Source: CAD feature listing. Evaluate the final solid. Frame: model axes, mm. A direction names the side the tool comes from. Round coordinates to 2 decimals unless told otherwise and drop trailing zeros. Loops run counter-clockwise (first coordinate to the right, second up) from the corner with the lowest first, then second, coordinate; pieces in that order, holes last.
(1) Section C-C, the plane y = 4.5. Return the cut outline in (x, z) (3 decimals), plus the area to 3 significant figures.
(2) Section A-A, the plane x = 0. Return the cut outline in (y, z), plus the area to 3 significant figures.
(3) Mould query, pull axis X, two halves, no side actions, for faces 1 (the flat face through (7, 0, -7)), 2 (the cylindrical face through (-9.874, 8.535, -9.663)), 3 (the cylindrical face through (9.777, 9.042, 9.758)). Classes: pulls with the +X half, pulls with the -X half, needs draft (parallel to the pull), parting line crosses it, or undercut.
(4) Material intervals for probe 1 along X at (y, z) = (8.2, 0); probe 2 along Y at (x, z) = (-0.75, -9); probe 3 along Z at (x, y) = (-14.75, 9), sorted ascending.
(5) Section B-B, the plane y = 10.25. Return the cut outline in (x, z).
(6) First-contact query: pin 1 Ø10 at (x, z) = (3.5, 0) entering from +Y; pin 2 Ø6 at (y, z) = (2.5, -9) entering from +X; pin 3 Ø9 at (x, z) = (0, 0) entering from -Y. Flat tips, straight axial feed; report the tip coordinate or a pass-through.
(7) Set-up query: faces 4 (the conical face through (-13.585, 11.16, 7.574)), 5 (the cylindrical face through (-5.776, 3.042, -8.602)). Return all of +Z, -Z, +X, -X, +Y, -Y with unobstructed straight access to the full face (end or side cutting, diameter ignored); none if empty.
```python
from build123d import *

# Parameters (mm, degrees)
SKETCH1_W                   = 21
SKETCH1_H                   = 21
BOSS_EXTRUDE1_DEPTH         = 12
CUT_EXTRUDE1_REACH          = 21.092
SKETCH2_R                   = 7.4
SKETCH3_W                   = 21
SKETCH3_H                   = 6
BOSS_EXTRUDE2_DEPTH         = 8.99
SKETCH4_W                   = 21
SKETCH4_H                   = 6
BOSS_EXTRUDE3_DEPTH         = 8.99
SKETCH5_R                   = 2.5
BOSS_EXTRUDE4_DEPTH         = 6
CUT_EXTRUDE2_REACH          = 24.937
SKETCH6_R                   = 2.6
CIRPATTERN1_COUNT           = 2
CIRPATTERN1_ANGLE           = 90
CIRPATTERN1_COPY_1_SKETCH_R = 2.5
CIRPATTERN1_COPY_1_DEPTH    = 6
CIRPATTERN1_COPY_2_REACH    = 24.937
CIRPATTERN1_COPY_2_SKETCH_R = 2.6
SKETCH7_W                   = 31.659066887
SKETCH7_H                   = 31.46982372
CUT_EXTRUDE3_DEPTH          = 11
FILLET1_R                   = 7
SKETCH9_R                   = 7.4
CUT_EXTRUDE4_DEPTH          = 11
CIRPATTERN2_COUNT           = 4
SKETCH10_R                  = 2
BOSS_EXTRUDE5_DEPTH         = 6
CIRPATTERN3_COUNT           = 4
CHAMFER1_SIZE               = 1
CHAMFER2_SIZE               = 1


with BuildPart() as part:
    # Sketch1 → Boss-Extrude1 (new body)
    with BuildSketch(Plane(origin=(0, 0, 0), x_dir=(1, 0, 0), z_dir=(0, 1, 0))):
        Rectangle(SKETCH1_W, SKETCH1_H)
    extrude(amount=BOSS_EXTRUDE1_DEPTH)

    # Sketch2 → Cut-Extrude1 (cut, up to next)
    with BuildSketch(Plane(origin=(0, 12, 0), x_dir=(1, 0, 0), z_dir=(0, 1, 0)), mode=Mode.PRIVATE) as cut_extrude1_sk1:
        with Locations(Location((0, 0, 0), (0, 0, 270))):
            Circle(SKETCH2_R)
    cut_extrude1_tool1 = extrude(cut_extrude1_sk1.sketch, amount=-CUT_EXTRUDE1_REACH, mode=Mode.PRIVATE) & part.part
    add(cut_extrude1_tool1.solids().sort_by_distance((0, 12, 0))[0], mode=Mode.SUBTRACT)

    # Sketch3 → Boss-Extrude2 (add)
    with BuildSketch(Plane.XY.offset(10.5)):
        with Locations((0, 3)):
            Rectangle(SKETCH3_W, SKETCH3_H)
    boss_extrude2 = extrude(amount=BOSS_EXTRUDE2_DEPTH)

    # Sketch4 → Boss-Extrude3 (add)
    with BuildSketch(Plane(origin=(0, 0, -10.5), x_dir=(-1, 0, 0), z_dir=(0, 0, -1))):
        with Locations((0, 9)):
            Rectangle(SKETCH4_W, SKETCH4_H)
    boss_extrude3 = extrude(amount=BOSS_EXTRUDE3_DEPTH)

    # Sketch5 → Boss-Extrude4 (add)
    with BuildSketch(Plane.XZ.offset(-6)):
        with Locations(Location((4, -14.995, 0), (0, 0, 90))):
            Circle(SKETCH5_R)
    boss_extrude4 = extrude(amount=BOSS_EXTRUDE4_DEPTH)

    # Sketch6 → Cut-Extrude2 (cut, up to next)
    with BuildSketch(Plane(origin=(0, 6, 0), x_dir=(1, 0, 0), z_dir=(0, 1, 0)), mode=Mode.PRIVATE) as cut_extrude2_sk1:
        with Locations(Location((4.5, -14.995, 0), (0, 0, 270))):
            Circle(SKETCH6_R)
    cut_extrude2_tool1 = extrude(cut_extrude2_sk1.sketch, amount=-CUT_EXTRUDE2_REACH, mode=Mode.PRIVATE) & part.part
    cut_extrude2 = cut_extrude2_tool1.solids().sort_by_distance((4.5, 6, 14.995))[0]
    add(cut_extrude2, mode=Mode.SUBTRACT)

    # Mirror1: Boss-Extrude4 across plane
    add(boss_extrude4.mirror(Plane(origin=(0, 0, 0), x_dir=(0, 0, 1), z_dir=(1, 0, 0))))

    # Mirror2: Cut-Extrude2 across plane
    add(cut_extrude2.mirror(Plane(origin=(0, 0, 0), x_dir=(0, 0, 1), z_dir=(1, 0, 0))), mode=Mode.SUBTRACT)

    # CirPattern1: Boss-Extrude2, Boss-Extrude3, Boss-Extrude4, Cut-Extrude2 ×2 about axis
    cirpattern1_axis = Axis((0, 0, 0), (0, 1, 0))
    add([boss_extrude2.rotate(cirpattern1_axis, i * CIRPATTERN1_ANGLE / (CIRPATTERN1_COUNT - 1)) for i in range(1, CIRPATTERN1_COUNT)])
    add([boss_extrude3.rotate(cirpattern1_axis, i * CIRPATTERN1_ANGLE / (CIRPATTERN1_COUNT - 1)) for i in range(1, CIRPATTERN1_COUNT)])
    add([boss_extrude4.rotate(cirpattern1_axis, i * CIRPATTERN1_ANGLE / (CIRPATTERN1_COUNT - 1)) for i in range(1, CIRPATTERN1_COUNT)])
    add([cut_extrude2.rotate(cirpattern1_axis, i * CIRPATTERN1_ANGLE / (CIRPATTERN1_COUNT - 1)) for i in range(1, CIRPATTERN1_COUNT)], mode=Mode.SUBTRACT)

    # CirPattern1 copy 1 sketch → CirPattern1 copy 1 (add)
    with BuildSketch(Plane(origin=(0, 6, 0), x_dir=(0, 0, 1), z_dir=(0, -1, 0))):
        with Locations((4, 14.995)):
            Circle(CIRPATTERN1_COPY_1_SKETCH_R)
    extrude(amount=CIRPATTERN1_COPY_1_DEPTH)

    # CirPattern1 copy 2 sketch → CirPattern1 copy 2 (cut, up to next)
    with BuildSketch(Plane.ZX.offset(6), mode=Mode.PRIVATE) as cirpattern1_copy_2_sk1:
        with Locations((4.5, 14.995)):
            Circle(CIRPATTERN1_COPY_2_SKETCH_R)
    cirpattern1_copy_2_tool1 = extrude(cirpattern1_copy_2_sk1.sketch, amount=-CIRPATTERN1_COPY_2_REACH, mode=Mode.PRIVATE) & part.part
    add(cirpattern1_copy_2_tool1.solids().sort_by_distance((14.995, 6, 4.5))[0], mode=Mode.SUBTRACT)

    # Sketch7 → Cut-Extrude3 (cut)
    with BuildSketch(Plane.XZ.offset(-6)):
        with Locations((5.329533444, 5.23491186)):
            Rectangle(SKETCH7_W, SKETCH7_H)
    extrude(amount=CUT_EXTRUDE3_DEPTH, mode=Mode.SUBTRACT)

    # Fillet1
    fillet1_edges = [part.edges().sort_by_distance(p)[0] for p in [
        (-10.5, 9, -10.5),
    ]]
    fillet(fillet1_edges, radius=FILLET1_R)

    # Sketch9 → Cut-Extrude4 (cut)
    with BuildSketch(Plane(origin=(0, 12, 0), x_dir=(1, 0, 0), z_dir=(0, 1, 0))):
        with Locations((-15, 15)):
            Circle(SKETCH9_R)
    cut_extrude4 = extrude(amount=-CUT_EXTRUDE4_DEPTH, mode=Mode.SUBTRACT)

    # CirPattern2: Cut-Extrude4 ×4 about axis
    cirpattern2_axis = Axis((0, 0, 0), (0, 1, 0))
    for i in range(1, CIRPATTERN2_COUNT):
        add(cut_extrude4.rotate(cirpattern2_axis, i * 360 / CIRPATTERN2_COUNT), mode=Mode.SUBTRACT)

    # Sketch10 → Boss-Extrude5 (add)
    with BuildSketch(Plane.XZ.offset(-6)):
        with Locations(Location((-7.25, 7.25, 0), (0, 0, 90))):
            Circle(SKETCH10_R)
    boss_extrude5 = extrude(amount=BOSS_EXTRUDE5_DEPTH)

    # CirPattern3: Boss-Extrude5 ×4 about axis
    cirpattern3_axis = Axis((0, 0, 0), (0, 1, 0))
    for i in range(1, CIRPATTERN3_COUNT):
        add(boss_extrude5.rotate(cirpattern3_axis, i * 360 / CIRPATTERN3_COUNT))

    # Chamfer1
    chamfer1_edges = [part.edges().sort_by_distance(p)[0] for p in [
        (0, 12, -7.4),
    ]]
    chamfer(chamfer1_edges, length=CHAMFER1_SIZE)

    # Chamfer2
    chamfer2_edges = [part.edges().sort_by_distance(p)[0] for p in [
        (-9.767409819, 12, -9.767409819),
        (7.664935028, 12, -14.02182729),
        (-14.02182729, 12, 7.664935028),
    ]]
    chamfer(chamfer2_edges, length=CHAMFER2_SIZE)


solid = part.part
```
Output values:
1. outline: circle Ø5 at (-14.995, -4); circle Ø5 at (-14.995, 4); circle Ø4 at (-7.25, -7.25); circle Ø4 at (-7.25, 7.25); circle Ø5 at (-4, -14.995); circle Ø5 at (4, -14.995); circle Ø4 at (7.25, -7.25); circle Ø4 at (7.25, 7.25)
1. area: 129 mm2
2. outline: (6, -19.49) - (12, -19.49) - (12, -8.4) - (11, -7.4) - (6, -7.4) - close; (6, 7.4) - (11, 7.4) - (12, 8.4) - (12, 10.5) - (6, 10.5) - close
2. area: 90.1 mm2
3. face 1: needs draft
3. face 2: undercut
3. face 3: pulls with the +X half
4. probe 1: x = -19.49 to -7.4, 7.4 to 10.5
4. probe 2: y = 6 to 12
4. probe 3: z = -7.6 to 7.6
5. outline: (-19.49, -9.12) arc R7.4 cw to (-9.12, -19.49) - (9.12, -19.49) arc R7.4 cw to (10.5, -9.13) - (10.5, 9.13) arc R7.4 cw to (9.13, 10.5) - (-9.13, 10.5) arc R7.4 cw to (-19.49, 9.12) - close; hole circle Ø14.8 at (0, 0)
6. pin 1: stops at y = 12
6. pin 2: stops at x = 9.25
6. pin 3: passes through
7. face 4: +Z, +Y
7. face 5: -Y
